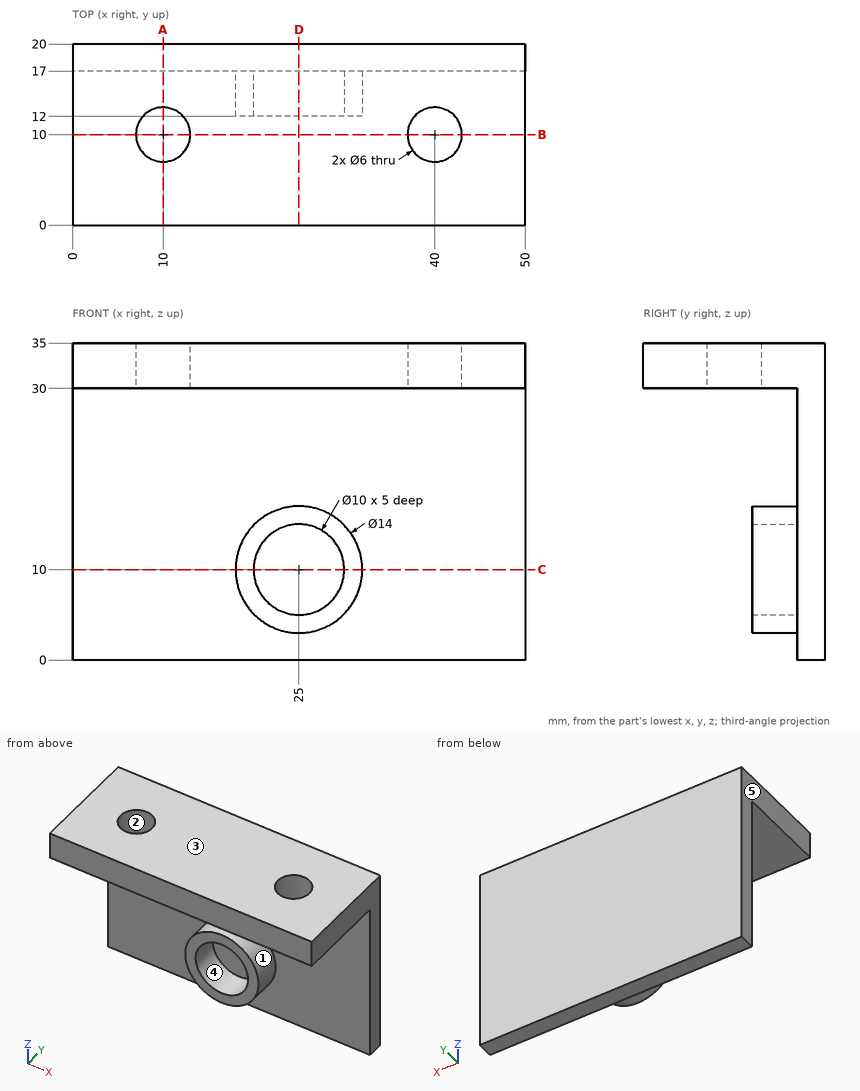
Check sheet for the drawn part. Datum: minimum x, y, z corner. Units: mm. A direction names the side the tool comes from. Round coordinates to 2 decimals unless told otherwise and drop trailing zeros. Loops run counter-clockwise (first coordinate to the right, second up) from the corner with the lowest first, then second, coordinate; pieces in that order, holes last.
Item 1: Cross-section at C-C on z = 10. Record the boundary of the cut face in (x, y), then the cut area to 3 significant figures.
Item 2: Gauge pin test, flat ends, axial feed: pin 1 (7 mm diameter, centred on x = 25.5, z = 9.5, fed in from -Y); pin 2 (7 mm diameter, centred on x = 10, y = 10, fed in from +Z); pin 3 (3 mm diameter, centred on x = 21.5, y = 9, fed in from -Z); pin 4 (6 mm diameter, centred on y = 13, z = 4.5, fed in from -X). Record the tip position at first contact, or that the pin passes through.
Item 3: Access from +Z, -Z, +X, -X, +Y, -Y to the whole of each face (thin tool, end or side, straight path). Record for the marked faces 1 and 2.
Item 4: Thickness scan on line 1 (Z direction, x = 25, y = 13.1); line 2 (Y direction, x = 10, z = 33.4); line 3 (Y direction, x = 44, z = 20). Record the ranges inside material, lowest first.
Item 5: Mould release check, pull along Z, two halves, no side actions. Record for the marked faces 3, 4 and 5: pulls with the +Z half, pulls with the -Z half, needs draft (parallel to the pull), parting line crosses it, or undercut.
Item 6: Cross-section at D-D on x = 25. Record the boundary of the cut face in (y, z), then the cut area to 3 significant figures.
Item 7: Cross-section at B-B on y = 10. Record the boundary of the cut face in (x, z), then the cut area to 3 significant figures.
Item 8: Cross-section at A-A on x = 10. Record the boundary of the cut face in (y, z), then the cut area to 3 significant figures.
Answer sheet:
1. outline: (0, 17) - (18, 17) - (18, 12) - (20, 12) - (20, 17) - (30, 17) - (30, 12) - (32, 12) - (32, 17) - (50, 17) - (50, 20) - (0, 20) - close
1. area: 170 mm2
2. pin 1: stops at y = 17
2. pin 2: stops at z = 35
2. pin 3: stops at z = 30
2. pin 4: stops at x = 18.46
3. face 1: -Y
3. face 2: +Z, -Z
4. line 1: z = 3 to 5, 15 to 17, 30 to 35
4. line 2: y = 0 to 7, 13 to 20
4. line 3: y = 17 to 20
5. face 3: pulls with the +Z half
5. face 4: undercut
5. face 5: needs draft
6. outline: (0, 30) - (17, 30) - (17, 17) - (12, 17) - (12, 15) - (17, 15) - (17, 5) - (12, 5) - (12, 3) - (17, 3) - (17, 0) - (20, 0) - (20, 35) - (0, 35) - close
6. area: 210 mm2
7. outline: (0, 30) - (7, 30) - (7, 35) - (0, 35) - close; (13, 30) - (37, 30) - (37, 35) - (13, 35) - close; (43, 30) - (50, 30) - (50, 35) - (43, 35) - close
7. area: 190 mm2
8. outline: (0, 30) - (7, 30) - (7, 35) - (0, 35) - close; (13, 30) - (17, 30) - (17, 0) - (20, 0) - (20, 35) - (13, 35) - close
8. area: 160 mm2
